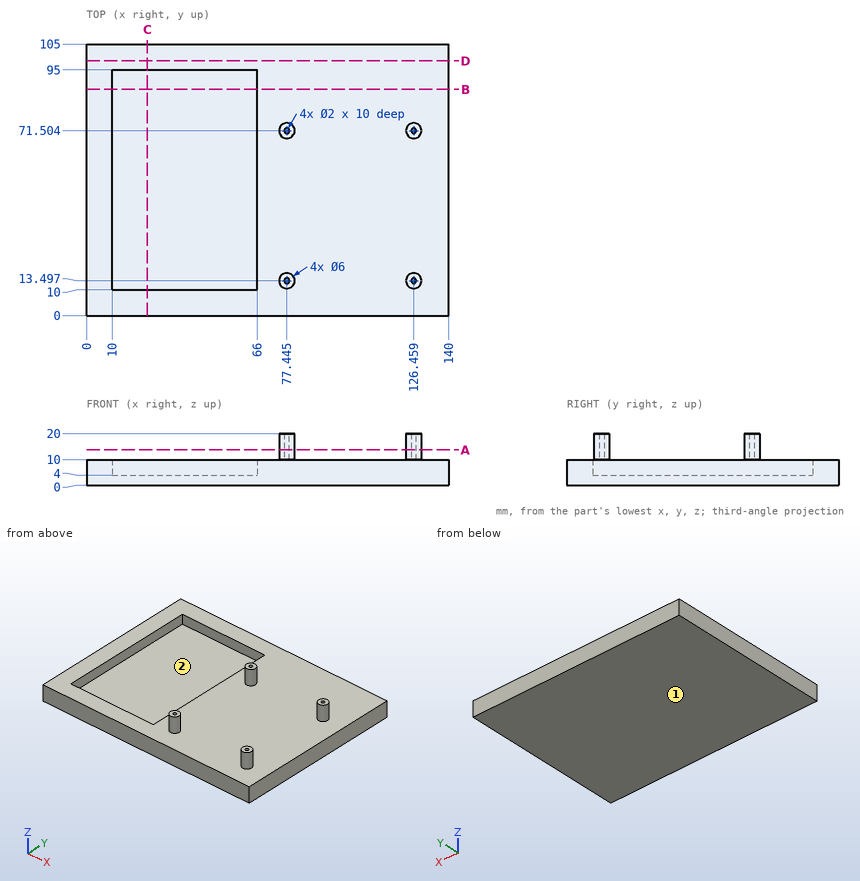
Source: three-view drawing plus pictorial views. Frame: mm from the lowest corner of the part. Coordinates: 2 decimals unless noted, no trailing zeros. Write each loop counter-clockwise with the first axis right and the second up, starting at its lowest first coordinate (ties: lowest second). Pieces come first, ordered by that corner, then holes. Notation, with made-up numbers: (65, 54.5) -> (110, 54.5) arc R23 cw to (110, 68.5) -> close; hole circle Ø9 at (-23, -9). An arc over 180 degrees is marked (long way). Write each question's results on one line, items separated by ' | '.
Item 1: Mould query, pull axis Y, two halves, no side actions, for the marked faces 1 and 2. Classes: +Y half, -Y half, draft (parallel to the pull), parting line (faces both ways), or undercut.
Conclusion:
face 1: draft | face 2: undercut
Item 2: Section query A-A on z = 13.75. Return loops of the section in (x, y) (1 decimal).
Conclusion:
outline: circle Ø6 at (77.4, 13.5); circle Ø6 at (77.4, 71.5); circle Ø6 at (126.5, 13.5); circle Ø6 at (126.5, 71.5); hole circle Ø2 at (77.4, 13.5); hole circle Ø2 at (77.4, 71.5); hole circle Ø2 at (126.5, 13.5); hole circle Ø2 at (126.5, 71.5)
Item 3: Section query D-D on y = 98.5. Return loops of the section in (x, z), plus the area to 3 significant figures.
Conclusion:
outline: (0, 0) -> (140, 0) -> (140, 10) -> (0, 10) -> close | area: 1,400 mm^2
Item 4: Pin query (flat end, axial travel): pin 1 Ø2 at (x, z) = (109.5, 6) entering from -Y; pin 2 Ø0.6 at (x, y) = (77, 13.5) entering from +Z; pin 3 Ø5 at (y, z) = (69.5, 13.5) entering from -X (1 decimal). Return the tip coordinate at first contact, or that it passes through.
Conclusion:
pin 1: stops at y = 0 | pin 2: stops at z = 10 | pin 3: stops at x = 74.4
Item 5: Section query B-B on y = 87.5. Return loops of the section in (x, z).
Conclusion:
outline: (0, 0) -> (140, 0) -> (140, 10) -> (66, 10) -> (66, 4) -> (10, 4) -> (10, 10) -> (0, 10) -> close
Item 6: Section query C-C on x = 23.5. Return loops of the section in (y, z), plus the area to 3 significant figures.
Conclusion:
outline: (0, 0) -> (105, 0) -> (105, 10) -> (95, 10) -> (95, 4) -> (10, 4) -> (10, 10) -> (0, 10) -> close | area: 540 mm^2
Item 7: Material intervals for probe 1 along X at (y, z) = (57, 8); probe 2 along Y at (x, z) = (27.5, 6); probe 3 along Z at (x, y) = (91, 64), sorted ascending.
Conclusion:
probe 1: x = 0 to 10, 66 to 140 | probe 2: y = 0 to 10, 95 to 105 | probe 3: z = 0 to 10
